For this review, use the dimensioned drawing (mm, ordinates from the lowest corner) and the shaded views. A direction names the side the tool comes from. Round coordinates to 2 decimals unless told otherwise and drop trailing zeros. Write each loop counter-clockwise with the first axis right and the second up, starting at its lowest first coordinate (ties: lowest second). Pieces come first, ordered by that corner, then holes. Notation, with made-up numbers: M -23,17.5 L 23,17.5 A15 ccw 23,28.5 Z; hole C 16.5,10.5 d4. An arc over 180 degrees is marked long. Answer in a Markdown table with one row per item.
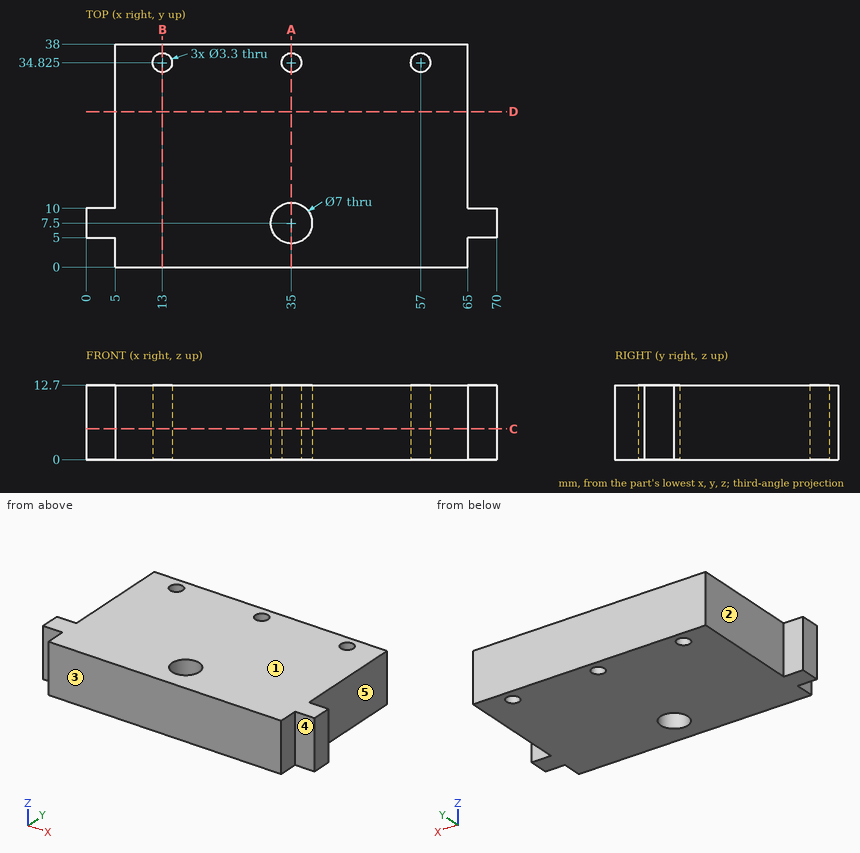
Q1. Take a section at D-D (y = 26.5). State the section outline as (x, z) points, then the cut area to 3 significant figures.
Found:
| item | result |
|---|---|
| outline | M 5,0 L 65,0 L 65,12.7 L 5,12.7 Z |
| area | 762 mm² |
Q2. Take a section at A-A (x = 35). State the section outline as (y, z) points (3 decimals), then the cut area to 3 significant figures.
Found:
| item | result |
|---|---|
| outline | M 0,0 L 4,0 L 4,12.7 L 0,12.7 Z; M 11,0 L 33.175,0 L 33.175,12.7 L 11,12.7 Z; M 36.475,0 L 38,0 L 38,12.7 L 36.475,12.7 Z |
| area | 352 mm² |
Q3. Take a section at B-B (x = 13). State the section outline as (y, z) points (3 decimals), then the cut area to 3 significant figures.
Found:
| item | result |
|---|---|
| outline | M 0,0 L 33.175,0 L 33.175,12.7 L 0,12.7 Z; M 36.475,0 L 38,0 L 38,12.7 L 36.475,12.7 Z |
| area | 441 mm² |
Q4. Insertion check: P1, Ø2.5, axis at x = 1.5, z = 5, coming from the -Y side; P2, Ø6.5, axis at x = 35, y = 7.5, coming from the +Z side; P3, Ø4, axis at y = 19.5, z = 8.5, coming from the +X side; P4, Ø2.5, axis at x = 1.5, z = 6.5, coming from the +Y side. Each pin has a flat end and moves straight along its axis. Give the tip position at first contact, or say it passes through.
Found:
| item | result |
|---|---|
| P1 | y = 5 |
| P2 | through |
| P3 | x = 65 |
| P4 | y = 10 |
Q5. Take a section at C-C (z = 5.25). State the section outline as (x, y) points (3 decimals).
Found:
| item | result |
|---|---|
| outline | M 0,5 L 5,5 L 5,0 L 65,0 L 65,5 L 70,5 L 70,10 L 65,10 L 65,38 L 5,38 L 5,10 L 0,10 Z; hole C 13,34.825 d3.3; hole C 35,7.5 d7; hole C 35,34.825 d3.3; hole C 57,34.825 d3.3 |
Q6. Machinability: for the marked faces 1, 2, 3, 4 and 5, which of the approach directions +Z, -Z, +X, -X, +Y, -Y give a long, thin tool a straight path to every point of the face, cutting with its end or side? Answer none if there is none.
Found:
| item | result |
|---|---|
| face 1 | +Z, +X, -X, +Y, -Y |
| face 2 | +Z, -Z, -X, +Y |
| face 3 | +Z, -Z, +X, -X, -Y |
| face 4 | +Z, -Z, +X, -Y |
| face 5 | +Z, -Z, +X, +Y |
Q7. For probe 1 along Y at (x, z) = (35, 6.5) (3 decimals); probe 2 along Y at (x, z) = (13, 6.75) (3 decimals); probe 3 along X at (y, z) = (34, 6.75), list the stretches that pass through material, from the lowest coordinate up.
Found:
| item | result |
|---|---|
| probe 1 | 0 to 4, 11 to 33.175, 36.475 to 38 |
| probe 2 | 0 to 33.175, 36.475 to 38 |
| probe 3 | 5 to 11.57, 14.43 to 33.57, 36.43 to 55.57, 58.43 to 65 |
